The listing builds one solid part. Answer for the finished solid, in the listing's coordinates (mm). Round coordinates to 2 decimals unless told otherwise and drop trailing zeros. Order: outer loops, then holes, each group sorted by start corner. A loop starts at its lowest first (then second) coordinate and runs counter-clockwise, first axis right, second up. Notation, with made-up numbers: (-27, -18) -> (20, -18) arc R21 cw to (20, 4) -> close; hole circle Ø2 at (12, -14.75). An arc over 180 degrees is marked (long way). Answer in a Markdown table with one row per item. Add a question column.
```python
from build123d import *

# Parameters (mm, degrees)
F0_W      = 540
F0_H      = 390
F1_DEPTH  = 10
F2_W      = 80
F2_H      = 80
F2_R      = 15
F3_DEPTH  = 10
F5_W      = 380
F5_H      = 80
F6_DEPTH  = 10
F7_DEPTH  = 25
F8_W      = 111.767
F8_H      = 26.2346411405
F9_DEPTH  = 25
F10_DEPTH = 130


with BuildPart() as f1:
    # F0 (on Front) → F1 (new body)
    with BuildSketch(Plane.XZ):
        Polygon((-575.5810141563, 243.9473703504), (-465.5810141563, -206.0526296496), (133.660423523, -206.0526296496), (243.660423523, 243.9473703504), (133.660423523, 243.9473703504), (-465.5810141563, 243.9473703504), align=None)
        with Locations((-166.339576477, 18.9473703504)):
            Rectangle(F0_W, F0_H, mode=Mode.SUBTRACT)
        Polygon((-495.5810141563, 43.0153865893), (-537.3643879646, 213.9473703504), (-495.5810141563, 213.9473703504), align=None, mode=Mode.SUBTRACT)
        Polygon((163.660423523, 213.9473703504), (205.4437973313, 213.9473703504), (163.660423523, 43.0153865893), align=None, mode=Mode.SUBTRACT)
    extrude(amount=F1_DEPTH)

    # F2 (on face) → F3 (join)
    with BuildSketch(Plane.XZ.offset(10)):
        with Locations((-396.339576477, 173.9473703504)):
            Rectangle(F2_W, F2_H)
        with Locations((-396.339576477, 198.0975481868)):
            Circle(F2_R, mode=Mode.SUBTRACT)
        with Locations((63.660423523, 173.9473703504)):
            Rectangle(F2_W, F2_H)
        with Locations((63.660423523, 198.0975481868)):
            Circle(F2_R, mode=Mode.SUBTRACT)
        with Locations((63.660423523, -136.0526296496)):
            Rectangle(F2_W, F2_H)
        with Locations((63.660423523, -136.0526296496)):
            Circle(F2_R, mode=Mode.SUBTRACT)
        with Locations((-396.339576477, -136.0526296496)):
            Rectangle(F2_W, F2_H)
        with Locations((-396.339576477, -136.0526296496)):
            Circle(F2_R, mode=Mode.SUBTRACT)
    extrude(amount=-F3_DEPTH)

    # F5 (on face) → F6 (join)
    with BuildSketch(Plane.XZ.offset(10)):
        with Locations((-166.339576477, 173.9473703504)):
            Rectangle(F5_W, F5_H)
    extrude(amount=-F6_DEPTH)

    # F4 (on face) → F7 (cut)
    with BuildSketch(Plane.XZ.offset(10)):
        Polygon((3.5932296524, 243.9473703504), (-339.0040903476, 243.9473703504), (-339.0040903476, 218.5033703504), (-286.9719266891, 218.5033703504), (3.5932296524, 218.5033703504), align=None)
    extrude(amount=-F7_DEPTH, mode=Mode.SUBTRACT)

    # F8 (on face) → F9 (cut)
    with BuildSketch(Plane.XZ.offset(10)):
        with Locations((-193.0365383425, 205.3860497801)):
            Rectangle(F8_W, F8_H)
    extrude(amount=-F9_DEPTH, mode=Mode.SUBTRACT)

    # F10 (add): a face of the model
    f10_faces = [f1.faces().sort_by_distance(p)[0] for p in [
        (-166.339576477, -5, 133.9473703504),
    ]]
    extrude(f10_faces, amount=F10_DEPTH)


solid = f1.part
```
Item 1: For a pull along Z with two mould halves and no side action, classify faces 1 (the face through (-172, 0, 72)), 2 (the face through (-521.35, -4.93, 22.1)), 3 (the face through (-516.18, -4.93, 127.28)) as released by +Z, released by -Z, zero draft, split by the parting line, or undercut.
Item 2: The part is cut by section B-B, the plane y = -6. State how many separate pieces and enclosed holes the cut face has, and give its area (3 significant figures).
Item 3: The part is cut by section A-A, the plane x = -235.5. Give the vertices of the cut face in (y, z), and give its area (3 significant figures).
Item 4: The part is cut by section C-C, the plane x = -397.5. Give the vertices of the cut face in (y, z).
Item 5: Flat-ended cylindrical pins translate along their axes: P1, Ø2, axis at y = -5.5, z = -42.5, coming from the +X side; P2, Ø3, axis at y = -3, z = 233, coming from the -X side; P3, Ø6, axis at y = -5, z = -93.5, coming from the +X side. Find the tip coordinate at first contact, or state that the pin passes through.
Item 6: Find the intervals of material crossed by probe 1 along Z at (x, y) = (-244.5, -5.5); probe 2 along Z at (x, y) = (83, -2.25); probe 3 along X at (y, z) = (-2.75, 44) (3 decimals), in increasing order. Write a range as [from, to].
Item 7: The part is cut by section D-D, the plane z = 84. Give the vertices of the cut face in (x, y).
Resolved:
| question | item | result |
|---|---|---|
| 1 | face 1 | zero draft |
| 1 | face 2 | released by -Z |
| 1 | face 3 | undercut |
| 2 | separate pieces | 1 |
| 2 | enclosed holes | 7 |
| 2 | area | 213,000 mm2 |
| 3 | outline | (-10, -206.05) -> (0, -206.05) -> (0, -176.05) -> (-10, -176.05) -> close; (-10, 3.95) -> (0, 3.95) -> (0, 192.27) -> (-10, 192.27) -> close |
| 3 | area | 2,180 mm2 |
| 4 | outline | (-10, -206.05) -> (0, -206.05) -> (0, -151.01) -> (-10, -151.01) -> close; (-10, -121.1) -> (0, -121.1) -> (0, -96.05) -> (-10, -96.05) -> close; (-10, 3.95) -> (0, 3.95) -> (0, 183.14) -> (-10, 183.14) -> close; (-10, 213.05) -> (0, 213.05) -> (0, 243.95) -> (-10, 243.95) -> close |
| 5 | P1 | x = 173.88 |
| 5 | P2 | x = -573.27 |
| 5 | P3 | x = 161.91 |
| 6 | probe 1 | [-206.05, -176.05], [3.95, 192.27] |
| 6 | probe 2 | [-206.05, -96.05], [3.95, 243.95] |
| 6 | probe 3 | [-526.705, -495.822], [-495.581, 163.66], [163.901, 194.784] |
| 7 | outline | (-536.48, -10) -> (-505.6, -10) -> (-505.6, 0) -> (-536.48, 0) -> close; (-495.58, -10) -> (163.66, -10) -> (163.66, 0) -> (-495.58, 0) -> close; (173.68, -10) -> (204.56, -10) -> (204.56, 0) -> (173.68, 0) -> close |
